Read the model definition and answer for the solid it produces. Units are mm, in the model's axes. A direction names the side the tool comes from. Give positions to 0.01 mm unless a question says otherwise; leave off trailing zeros. Write each loop counter-clockwise with the first axis right and the second up, starting at its lowest first coordinate (ties: lowest second). Pieces come first, ordered by that corner, then holes.
```python
from build123d import *

# Parameters (mm, degrees)
F1_DEPTH = 63.5
F2_DEPTH = 25.4
F3_DEPTH = 8.255


with BuildPart() as f1:
    # F0 (on Front) → F1 (new body, symmetric)
    with BuildSketch(Plane.XZ):
        Polygon((-41.275, -9.525), (41.275, -9.525), (41.275, 9.525), (22.225, 9.525), (-41.275, 9.525), align=None)
    extrude(amount=F1_DEPTH, both=True)

    # F0 (on Front) → F2 (join, symmetric)
    with BuildSketch(Plane.XZ):
        with BuildLine():
            Line((22.225, 9.525), (41.275, 9.525))
            Line((41.275, 9.525), (41.275, 27.051))
            ThreePointArc((41.275, 27.051), (44.920476, 37.172974), (54.182636, 42.646204))
            Line((54.182636, 42.646204), (54.182636, 61.84799))
            add(Edge.make_bspline(
                [(54.096802, 61.842286), (54.125427, 61.844206), (54.154038, 61.846108), (54.182636, 61.84799)],
                knots=[108.458628, 108.458628, 108.458628, 108.458628, 108.543428, 108.543428, 108.543428, 108.543428], degree=3))
            ThreePointArc((54.096802, 61.842286), (31.397441, 50.642552), (22.225, 27.051))
            Line((22.225, 27.051), (22.225, 9.525))
        make_face()
        with BuildLine():
            Line((54.182636, 61.84799), (54.182636, 42.646204))
            ThreePointArc((54.182636, 42.646204), (55.659737, 42.855896), (57.15, 42.926))
            Line((57.15, 42.926), (73.837688, 42.926))
            Line((73.837688, 42.926), (79.582636, 42.926))
            Line((79.582636, 42.926), (79.582636, 61.976))
            Line((79.582636, 61.976), (73.837688, 61.976))
            Line((73.837688, 61.976), (57.15, 61.976))
            add(Edge.make_bspline(
                [(54.182636, 61.84799), (55.189281, 61.914258), (56.178968, 61.957255), (57.15, 61.976)],
                knots=[108.543428, 108.543428, 108.543428, 108.543428, 111.528418, 111.528418, 111.528418, 111.528418], degree=3))
        make_face()
    extrude(amount=F2_DEPTH, both=True)

    # F0 (on Front) → F3 (join, symmetric)
    with BuildSketch(Plane.XZ):
        with BuildLine():
            add(Edge.make_bspline(
                [(-41.275, 9.525), (-41.449575, 26.246032), (17.485724, 59.386473), (54.096802, 61.842286)],
                knots=[0, 0, 0, 0, 108.458628, 108.458628, 108.458628, 108.458628], degree=3))
            Line((-41.275, 9.525), (22.225, 9.525))
            Line((22.225, 9.525), (22.225, 27.051))
            ThreePointArc((22.225, 27.051), (31.397441, 50.642552), (54.096802, 61.842286))
        make_face()
    extrude(amount=F3_DEPTH, both=True)

    # F0 (on Front) → F4 (revolve)
    with BuildSketch(Plane.XZ):
        Polygon((79.582636, 42.926), (79.582636, 38.1), (104.982636, 38.1), (104.982636, 66.675), (79.582636, 66.675), (79.582636, 61.976), align=None)
    revolve(axis=Axis((79.582636, 0, 50.038), (0, 0, -1)))


solid = f1.part
```
Item 1: Which of the six approach directions +Z, -Z, +X, -X, +Y, -Y give full straight-line access (tool end or side, diameter ignored) to faces 1 (the flat face through (44, 25.4, 42)), 2 (the flat face through (22.225, -17, 18)), 3 (the flat face through (63, 22, 61.976)), 4 (the flat face through (80, 0, 38.1))?
Result set:
face 1: +Z, +X, -X, +Y
face 2: +Z, -X, -Y
face 3: +Z, -X, +Y
face 4: -Z, +X, +Y, -Y
Item 2: Each of these flat-tipped pins is pushed along its axis until it touches: pin 1 Ø16.5 at (x, y) = (-0.5, 31) entering from +Z (3 decimals); pin 2 Ø4 at (x, y) = (23.5, -22.5) entering from +Z; pin 3 Ø6 at (x, z) = (19, 39) entering from +Y (3 decimals). Where does it stop, or does it pass through?
Result set:
pin 1: stops at z = 9.525
pin 2: stops at z = 41.82
pin 3: stops at y = 8.255
Item 3: Determine the mould class of faces 5 (the flat face through (22.225, 17, 18)), 6 (the flat face through (-1, -1, -9.525)), 7 (the flat face through (62, -22, 42.926)) for opening direction X: pulls with the +X half, pulls with the -X half, needs draft (parallel to the pull), parting line crosses it, or undercut.
Result set:
face 5: pulls with the -X half
face 6: needs draft
face 7: undercut
Item 4: Section A-A (x = 86) is taken. Write down the section's boundary in (y, z) (3 decimals), and give its area (3 significant figures).
Result set:
outline: (-24.576, 38.1) - (24.576, 38.1) - (24.576, 66.675) - (-24.576, 66.675) - close
area: 1,400 mm2
Item 5: Find the intervals of material crossed by line 1 along X through (y, z) = (-18.5, 1) (3 decimals); line 2 along Y through (x, z) = (-8.5, 26.5) (3 decimals); line 3 along Z through (x, y) = (-32, -16.5) (3 decimals), in increasing order.
Result set:
line 1: x = -41.275 to 41.275
line 2: y = -8.255 to 8.255
line 3: z = -9.525 to 9.525
Item 6: Section B-B (y = 30) is taken. Write down the section's boundary in (x, z) (3 decimals).
Result set:
outline: (-41.275, -9.525) - (41.275, -9.525) - (41.275, 9.525) - (-41.275, 9.525) - close
